from build123d import *

# Parameters (mm, degrees)
F0_R     = 1.75
F1_DEPTH = 10


with BuildPart() as f1:
    # F0 (on Top) → F1 (new body)
    with BuildSketch(Plane.XY):
        with BuildLine():
            Line((25, 21), (-25, 21))
            Line((-25, 21), (-25, -21))
            Line((-25, -21), (-9, -21))
            Line((-9, -21), (-9, -6.324555))
            ThreePointArc((-9, -6.324555), (0, 11), (9, -6.324555))
            Line((9, -6.324555), (9, -21))
            Line((9, -21), (25, -21))
            Line((25, -21), (25, 21))
        make_face()
        with Locations((-15.5, -15.5)):
            Circle(F0_R, mode=Mode.SUBTRACT)
        with Locations((15.5, -15.5)):
            Circle(F0_R, mode=Mode.SUBTRACT)
        with Locations((-15.5, 15.5)):
            Circle(F0_R, mode=Mode.SUBTRACT)
        with Locations((15.5, 15.5)):
            Circle(F0_R, mode=Mode.SUBTRACT)
    extrude(amount=F1_DEPTH)


solid = f1.part
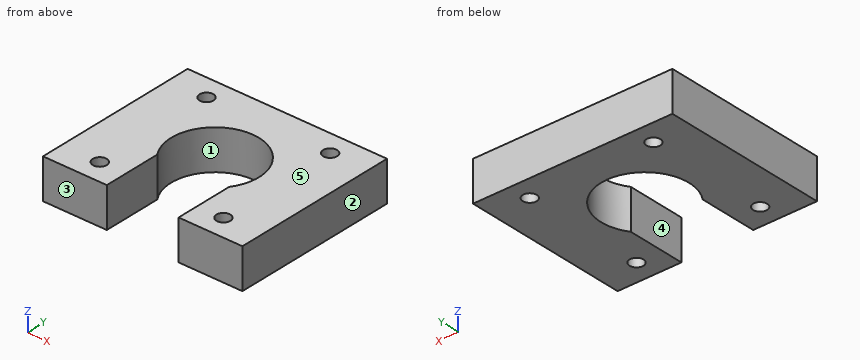
Can you work these out from the model? Positions are in its coordinate system, mm. Face numbers are marked on the shaded views. A direction names the side the tool comes from. Round coordinates to 2 decimals unless told otherwise and drop trailing zeros. Write each loop counter-clockwise with the first axis right and the second up, starting at its lowest first coordinate (ties: lowest second). Pieces come first, ordered by that corner, then holes. Notation, with made-up numbers: (17.25, -4.75) -> (28.25, -4.75) arc R12 ccw to (28.25, 11.25) -> close; hole circle Ø11 at (6.25, 23). An arc over 180 degrees is marked (long way). Use one line per item in the form item = value. Start each with the question number.
Q1. Imagine slicing it at C-C (x = -15.5). Please give me the cut outline in (y, z).
Q2. Imagine slicing it at B-B (y = 15.5). Please give me the cut outline in (x, z).
Q3. Imagine slicing it at D-D (z = 8.5). Please give me the cut outline in (x, y), then the cut area to 3 significant figures.
Q4. We'd pull the mould along Y, two halves only. Please class the marked faces 1, 2 and 3: +Y half, -Y half, draft (parallel to the pull), parting line (faces both ways), or undercut.
Q5. If I drill on probe 1 along Y at (x, z) = (-15.5, 3.25); probe 2 along X at (y, z) = (-10, 7.5); probe 3 along X at (y, z) = (0.5, 7.5), over which ranges is the centre line in solid material (lowest first)? Write a range as [from, to].
Q6. Which directions (+Z, -Z, +X, -X, +Y, -Y) give clear straight access to the entire face, cutting with the end or side of a thin tool? Please do the marked faces 4 and 5.
Q7. I'm going to push a flat-ended pin straight in: P1, Ø1.5, axis at x = -6, z = 6, coming from the -Y side. Where does the tip first touch, or does it pass through?
Q8. Imagine slicing it at A-A (y = -11). Please give me the cut outline in (x, z), then the cut area to 3 significant figures.
Worked out:
q1.outline = (-21, 0) -> (-17.25, 0) -> (-17.25, 10) -> (-21, 10) -> close; (-13.75, 0) -> (13.75, 0) -> (13.75, 10) -> (-13.75, 10) -> close; (17.25, 0) -> (21, 0) -> (21, 10) -> (17.25, 10) -> close
q2.outline = (-25, 0) -> (-17.25, 0) -> (-17.25, 10) -> (-25, 10) -> close; (-13.75, 0) -> (13.75, 0) -> (13.75, 10) -> (-13.75, 10) -> close; (17.25, 0) -> (25, 0) -> (25, 10) -> (17.25, 10) -> close
q3.outline = (-25, -21) -> (-9, -21) -> (-9, -6.32) arc R11 cw (long way) to (9, -6.32) -> (9, -21) -> (25, -21) -> (25, 21) -> (-25, 21) -> close; hole circle Ø3.5 at (-15.5, -15.5); hole circle Ø3.5 at (-15.5, 15.5); hole circle Ø3.5 at (15.5, -15.5); hole circle Ø3.5 at (15.5, 15.5)
q3.area = 1,480 mm^2
q4.face_1 = undercut
q4.face_2 = draft
q4.face_3 = -Y half
q5.probe_1 = [-21, -17.25], [-13.75, 13.75], [17.25, 21]
q5.probe_2 = [-25, -9], [9, 25]
q5.probe_3 = [-25, -10.99], [10.99, 25]
q6.face_4 = +Z, -Z, -Y
q6.face_5 = +Z, +X, -X, +Y, -Y
q7.P1 = 8.69
q8.outline = (-25, 0) -> (-9, 0) -> (-9, 10) -> (-25, 10) -> close; (9, 0) -> (25, 0) -> (25, 10) -> (9, 10) -> close
q8.area = 320 mm^2
